Autodesk Inventor part; units mm, degrees
ref_plane "YZ Plane" through (0, 0, 0) normal (1, 0, 0) x (0, 1, 0)
ref_plane "XZ Plane" through (0, 0, 0) normal (0, 1, 0) x (-1, 0, 0)
ref_plane "XY Plane" through (0, 0, 0) normal (0, 0, 1) x (1, 0, 0)
sketch "Эскиз1" plane through (0, 0, 0) normal (1, 0, 0) x (0, 1, 0)
  circle A0 centre (-6.0133, 48.1994) radius 2.75
  circle A1 centre (-6.0133, -0.8006) radius 2.75
  line L0 (-13.0133, 61.1994) -> (-13.0133, -18.8006)
  line L1 (38.9867, 61.1994) -> (-13.0133, 61.1994)
  line L2 (33.9867, -18.8006) -> (-13.0133, -18.8006)
  line L3 (-0.0133, 61.1994) -> (-0.0133, -18.8006)
  point P0 (0, 0)
  dimension "d0" = 13
extrude "Выдавливание1" add sketch "Эскиз1" against normal blind 10
sketch "Эскиз2" plane through (0, -13.0133, 61.1994) normal (0, 0, 1) x (1, 0, 0)
  line L0 (-55.25, 38) -> (-55.25, 36)
  line L1 (-10, 13) -> (-10, 0)
  line L2 (-10, 0) -> (-55.25, 36)
  line L3 (0, 13) -> (-10, 13)
  line L4 (-10, 13) -> (-42.25, 36)
  line L5 (-55.25, 36) -> (-42.25, 36)
  point P0 (0, 13.0133)
  dimension "d3" = 13
  dimension "d4" = 13
extrude "Выдавливание2" add sketch "Эскиз2" against normal up to surface (80 mm away)
sketch "Эскиз3" plane through (0, -13.0133, 61.1994) normal (0, 0, 1) x (1, 0, 0)
  line L0 (0, 13) -> (0, 0)
  line L1 (0, 13) -> (0, 36)
  line L2 (-10, 13) -> (-42.25, 36)
  line L3 (0, 36) -> (-42.25, 36)
  line L4 (0, 13) -> (-10, 13)
  point P0 (0, 13.0133)
extrude "Выдавливание3" add sketch "Эскиз3" against normal blind 4
sketch "Эскиз4" plane through (-10, -6.0133, 48.1994) normal (1, 0, 0) x (0, 0, -1)
  circle A0 centre (49, 0) radius 2.75
  circle A1 centre (0, 0) radius 2.75
  point P0 (48.1994, 6.0133)
extrude "Выдавливание4" cut sketch "Эскиз4" against normal through all
ref_plane "РабПлоскость1" through (-10, -13.0133, 61.1994) normal (1, 0, 0) x (0, 0, 1)
sketch "Эскиз5" plane through (-10, -13.0133, 61.1994) normal (1, 0, 0) x (0, 0, 1)
  circle A0 centre (-13, -7) radius 2.75
  circle A1 centre (-62, -7) radius 2.75
  circle A2 centre (-13, -7) radius 2.75
  circle A3 centre (-13, -7) radius 5
  circle A4 centre (-62, -7) radius 5
  point P0 (-61.1994, -13.0133)
  dimension "d12" = 10
  dimension "d13" = 10
extrude "Выдавливание5" cut sketch "Эскиз5" against normal through all contours A0 | A1 | A3 | A4
move faces "Перенос2" translate (0, 0, -40) faces at (-35.8333, 10.9867, -18.8006)
sketch "Эскиз6" plane through (0, -13.0133, -58.8006) normal (0, 0, -1) x (-1, 0, 0)
  line L0 (42.25, 36) -> (10, 13)
  line L1 (42.25, 36) -> (0, 36)
  line L2 (0, 36) -> (0, 13)
  line L3 (10, 13) -> (0, 13)
  point P0 (0, 13.0133)
extrude "Выдавливание6" add sketch "Эскиз6" against normal blind 4
equation "\"d4\" = d3"
properties part number "000.001.007 - Накладка"
Here's how the part is built. I have some questions about the finished solid (model axes, mm). A direction names the side the tool comes from. Coordinates: 2 decimals unless noted, no trailing zeros. Order: outer loops, then holes, each group sorted by start corner. A loop starts at its lowest first (then second) coordinate and runs counter-clockwise, first axis right, second up.
1) Imagine slicing it at B-B on x = -8. List the corners of the cut face in (y, z) for me, and give its area (3 significant figures).
2) I need wall thicknesses on line 1 (Z direction, x = -6.5, y = 8.5); line 2 (Z direction, x = -16, y = -8); line 3 (Y direction, x = -6, z = -6). Which ranges of each line are inside material? Lowest first, please.
3) Imagine slicing it at A-A on z = -7. List the corners of the cut face in (x, y) for me.
4) Imagine slicing it at C-C on y = 15. List the corners of the cut face in (x, z) for me.
5) Will these pins go through, and if not, where does the flat tip stop? pin 1 (16 mm diameter, centred on y = -6.01, z = -0.8, fed in from -X); pin 2 (4 mm diameter, centred on y = 8.5, z = -19, fed in from +X); pin 3 (3 mm diameter, centred on x = -4.5, z = 0.5, fed in from +Y).
6) Which directions (+Z, -Z, +X, -X, +Y, -Y) give clear straight access to the entire face, cutting with the end or side of a thin tool? Please do faces 5 (the face through (-5, -13.013, 2)), 6 (the face through (-25.899, 11.326, 1.983)), 7 (the face through (-15.77, -1.13, -1.88)).
7) We'd pull the mould along Y, two halves only. Please class faces 1 (the face through (-4.93, -8.76, -0.68)), 2 (the face through (-32.308, 4.735, 2.039)), 3 (the face through (-21, 9, -58.801)), 4 (the face through (-4.93, -6.371, 50.926)): +Y half, -Y half, draft (parallel to the pull), parting line (faces both ways), or undercut.
8) Imagine slicing it at D-D on x = -17. List the corners of the cut face in (y, z) for me, and give its area (3 significant figures).
Response values:
1. outline: (-13.01, -58.8) - (22.99, -58.8) - (22.99, -54.8) - (-0.01, -54.8) - (-0.01, 57.2) - (22.99, 57.2) - (22.99, 61.2) - (-13.01, 61.2) - close; hole circle Ø5.5 at (-6.01, -0.8); hole circle Ø5.5 at (-6.01, 48.2)
1. area: 1,700 mm2
2. line 1: z = -58.8 to -54.8, 57.2 to 61.2
2. line 2: z = -58.8 to -5.39, 3.79 to 43.61, 52.79 to 61.2
2. line 3: y = -13.01 to -0.01
3. outline: (-55.25, 22.99) - (-10, -13.01) - (0, -13.01) - (0, -0.01) - (-10, -0.01) - (-42.25, 22.99) - close
4. outline: (-45.21, -58.8) - (0, -58.8) - (0, -54.8) - (-31.05, -54.8) - (-31.05, 57.2) - (0, 57.2) - (0, 61.2) - (-45.21, 61.2) - close
5. pin 1: stops at x = -28.86
5. pin 2: stops at x = -19.13
5. pin 3: stops at y = -0.01
6. face 5: +Z, -Z, +X, -X, -Y
6. face 6: +X, +Y
6. face 7: -X
7. face 1: undercut
7. face 2: -Y half
7. face 3: draft
7. face 4: undercut
8. outline: (-7.44, -58.8) - (22.99, -58.8) - (22.99, -54.8) - (4.98, -54.8) - (4.98, 57.2) - (22.99, 57.2) - (22.99, 61.2) - (-7.44, 61.2) - (-7.44, 52.99) arc R5 cw (long way) to (-7.44, 43.41) - (-7.44, 3.99) arc R5 cw (long way) to (-7.44, -5.59) - close
8. area: 1,530 mm2
